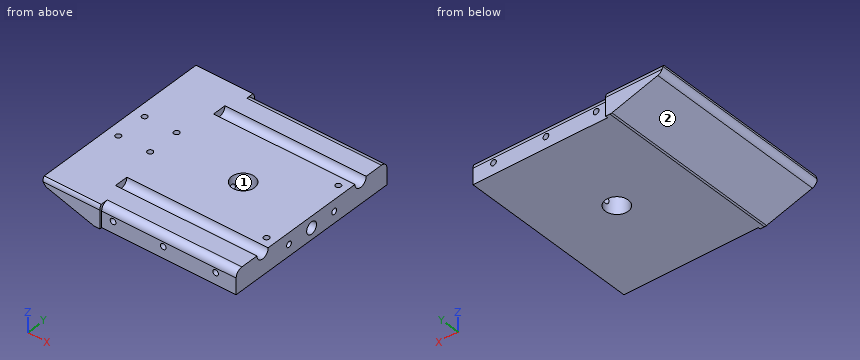
```python
from build123d import *

# Parameters (mm, degrees)
CYLINDER284_R          = 3
CYLINDER284_DEPTH      = 62
CYLINDER285_R          = 3
CYLINDER285_DEPTH      = 62
CYLINDER280_R          = 1.2
CYLINDER280_DEPTH      = 4
CYLINDER281_R          = 1.2
CYLINDER281_DEPTH      = 4
CYLINDER282_R          = 1.2
CYLINDER282_DEPTH      = 8
CYLINDER283_R          = 1.2
CYLINDER283_DEPTH      = 8
CYLINDER453_R          = 1.2
CYLINDER453_DEPTH      = 4
CYLINDER452_R          = 1.2
CYLINDER452_DEPTH      = 4
CYLINDER457_R          = 1.25
CYLINDER457_DEPTH      = 15
CYLINDER456_R          = 1.25
CYLINDER456_DEPTH      = 15
BOX301_W               = 25
BOX301_H               = 82
BOX301_DEPTH           = 1
CYLINDER278_R          = 1.25
CYLINDER278_DEPTH      = 15
CYLINDER277_R          = 1.25
CYLINDER277_DEPTH      = 15
CYLINDER279_R          = 1.25
CYLINDER279_DEPTH      = 15
CYLINDER272_R          = 1.6
CYLINDER272_DEPTH      = 41
CYLINDER274_R          = 2.6
CYLINDER274_DEPTH      = 20
CYLINDER273_R          = 1.4
CYLINDER273_DEPTH      = 51
CYLINDER286_R          = 1.25
CYLINDER286_DEPTH      = 15
CYLINDER287_R          = 1.25
CYLINDER287_DEPTH      = 15
CYLINDER288_R          = 1.25
CYLINDER288_DEPTH      = 15
CYLINDER271_R          = 5
CYLINDER271_DEPTH      = 19
BOX215_W               = 30
BOX215_H               = 82
BOX215_DEPTH           = 10
BOX215_PLACEMENT_ANGLE = 17
BOX214_W               = 25
BOX214_H               = 62
BOX214_DEPTH           = 1.5
BOX213_W               = 25
BOX213_H               = 82
BOX213_DEPTH           = 11
FILLET085_R            = 3
BOX212_W               = 60
BOX212_H               = 80
BOX212_DEPTH           = 10
FILLET084_R            = 3
FILLET086_R            = 3


with BuildPart() as cylinder284:
    # Cylinder284 → Cylinder284 (new body)
    with BuildSketch(Plane(origin=(67, 5, 19), x_dir=(0, 0, -1), z_dir=(1, 0, 0))):
        Circle(CYLINDER284_R)
    extrude(amount=CYLINDER284_DEPTH)


with BuildPart() as fusion252:
    # Cylinder285 → Cylinder285 (new body)
    with BuildSketch(Plane(origin=(67, 57, 19), x_dir=(0, 0, -1), z_dir=(1, 0, 0))):
        Circle(CYLINDER285_R)
    extrude(amount=CYLINDER285_DEPTH)

    # Fusion252: union Cylinder284
    add(cylinder284.part)


with BuildPart() as cylinder280:
    # Cylinder280 → Cylinder280 (new body)
    with BuildSketch(Plane(origin=(50, 24, 15), x_dir=(1, 0, 0), z_dir=(0, 0, 1))):
        Circle(CYLINDER280_R)
    extrude(amount=CYLINDER280_DEPTH)


with BuildPart() as cylinder281:
    # Cylinder281 → Cylinder281 (new body)
    with BuildSketch(Plane(origin=(50, 38, 15), x_dir=(1, 0, 0), z_dir=(0, 0, 1))):
        Circle(CYLINDER281_R)
    extrude(amount=CYLINDER281_DEPTH)


with BuildPart() as cylinder282:
    # Cylinder282 → Cylinder282 (new body)
    with BuildSketch(Plane(origin=(64, 24, 11), x_dir=(1, 0, 0), z_dir=(0, 0, 1))):
        Circle(CYLINDER282_R)
    extrude(amount=CYLINDER282_DEPTH)


with BuildPart() as cylinder283:
    # Cylinder283 → Cylinder283 (new body)
    with BuildSketch(Plane(origin=(64, 38, 11), x_dir=(1, 0, 0), z_dir=(0, 0, 1))):
        Circle(CYLINDER283_R)
    extrude(amount=CYLINDER283_DEPTH)


with BuildPart() as cylinder453:
    # Cylinder453 → Cylinder453 (new body)
    with BuildSketch(Plane(origin=(125, 12, 15), x_dir=(1, 0, 0), z_dir=(0, 0, 1))):
        Circle(CYLINDER453_R)
    extrude(amount=CYLINDER453_DEPTH)


with BuildPart() as fusion406:
    # Cylinder452 → Cylinder452 (new body)
    with BuildSketch(Plane(origin=(125, 50, 15), x_dir=(1, 0, 0), z_dir=(0, 0, 1))):
        Circle(CYLINDER452_R)
    extrude(amount=CYLINDER452_DEPTH)

    # Fusion406: union Cylinder280, Cylinder281, Cylinder282, Cylinder283, Cylinder453
    add(cylinder280.part)
    add(cylinder281.part)
    add(cylinder282.part)
    add(cylinder283.part)
    add(cylinder453.part)


with BuildPart() as cylinder457:
    # Cylinder457 → Cylinder457 (new body)
    with BuildSketch(Plane(origin=(80, 43, 14), x_dir=(0, 0, -1), z_dir=(1, 0, 0))):
        Circle(CYLINDER457_R)
    extrude(amount=CYLINDER457_DEPTH)


with BuildPart() as fusion414:
    # Cylinder456 → Cylinder456 (new body)
    with BuildSketch(Plane(origin=(80, 19, 14), x_dir=(0, 0, -1), z_dir=(1, 0, 0))):
        Circle(CYLINDER456_R)
    extrude(amount=CYLINDER456_DEPTH)

    # Fusion413: union Cylinder457
    add(cylinder457.part)


with BuildPart() as fusion414_1:
    # Fusion413 placement: moved
    add(fusion414.part.moved(Location((34, 0, 0))))

    # Fusion414: union Fusion252, Fusion406
    add(fusion252.part)
    add(fusion406.part)


with BuildPart() as cube372:
    # Box301 → Box301 (new body)
    with BuildSketch(Plane(origin=(45, -10, 19), x_dir=(1, 0, 0), z_dir=(0, 0, 1))):
        with Locations((12.5, 41)):
            Rectangle(BOX301_W, BOX301_H)
    extrude(amount=BOX301_DEPTH)


with BuildPart() as cylinder278:
    # Cylinder278 → Cylinder278 (new body)
    with BuildSketch(Plane(origin=(6, 15, 14), x_dir=(1, 0, 0), z_dir=(0, -1, 0))):
        Circle(CYLINDER278_R)
    extrude(amount=CYLINDER278_DEPTH)


with BuildPart() as cylinder277:
    # Cylinder277 → Cylinder277 (new body)
    with BuildSketch(Plane(origin=(28, 15, 14), x_dir=(1, 0, 0), z_dir=(0, -1, 0))):
        Circle(CYLINDER277_R)
    extrude(amount=CYLINDER277_DEPTH)


with BuildPart() as fusion246:
    # Cylinder279 → Cylinder279 (new body)
    with BuildSketch(Plane(origin=(51, 15, 14), x_dir=(1, 0, 0), z_dir=(0, -1, 0))):
        Circle(CYLINDER279_R)
    extrude(amount=CYLINDER279_DEPTH)

    # Fusion246: union Cylinder278, Cylinder277
    add(cylinder278.part)
    add(cylinder277.part)


with BuildPart() as fusion246_1:
    # Fusion246 placement: moved
    add(fusion246.part.moved(Location((0, 56, 0))))


with BuildPart() as cylinder272:
    # Cylinder272 → Cylinder272 (new body)
    with BuildSketch(Plane(origin=(20, 31, 10), x_dir=(0, 0, -1), z_dir=(1, 0, 0))):
        Circle(CYLINDER272_R)
    extrude(amount=CYLINDER272_DEPTH)


with BuildPart() as cylinder274:
    # Cylinder274 → Cylinder274 (new body)
    with BuildSketch(Plane(origin=(41, 31, 10), x_dir=(0, 0, -1), z_dir=(1, 0, 0))):
        Circle(CYLINDER274_R)
    extrude(amount=CYLINDER274_DEPTH)


with BuildPart() as fusion249:
    # Cylinder273 → Cylinder273 (new body)
    with BuildSketch(Plane(origin=(10, 31, 10), x_dir=(0, 0, -1), z_dir=(1, 0, 0))):
        Circle(CYLINDER273_R)
    extrude(amount=CYLINDER273_DEPTH)

    # Fusion249: union Cylinder272, Cylinder274
    add(cylinder272.part)
    add(cylinder274.part)


with BuildPart() as fusion249_1:
    # Fusion249 placement: moved
    add(fusion249.part.moved(Location((-1, 0, 4))))


with BuildPart() as cylinder286:
    # Cylinder286 → Cylinder286 (new body)
    with BuildSketch(Plane(origin=(6, 15, 14), x_dir=(1, 0, 0), z_dir=(0, -1, 0))):
        Circle(CYLINDER286_R)
    extrude(amount=CYLINDER286_DEPTH)


with BuildPart() as cylinder287:
    # Cylinder287 → Cylinder287 (new body)
    with BuildSketch(Plane(origin=(28, 15, 14), x_dir=(1, 0, 0), z_dir=(0, -1, 0))):
        Circle(CYLINDER287_R)
    extrude(amount=CYLINDER287_DEPTH)


with BuildPart() as fusion254:
    # Cylinder288 → Cylinder288 (new body)
    with BuildSketch(Plane(origin=(51, 15, 14), x_dir=(1, 0, 0), z_dir=(0, -1, 0))):
        Circle(CYLINDER288_R)
    extrude(amount=CYLINDER288_DEPTH)

    # Fusion254: union Cylinder286, Cylinder287
    add(cylinder286.part)
    add(cylinder287.part)


with BuildPart() as fusion254_1:
    # Fusion254 placement: moved
    add(fusion254.part.moved(Location((0, -9, 0))))


with BuildPart() as fusion255:
    # Cylinder271 → Cylinder271 (new body)
    with BuildSketch(Plane(origin=(30, 31, 6), x_dir=(1, 0, 0), z_dir=(0, 0, 1))):
        Circle(CYLINDER271_R)
    extrude(amount=CYLINDER271_DEPTH)

    # Fusion255: union Fusion246, Fusion249, Fusion254
    add(fusion246_1.part)
    add(fusion249_1.part)
    add(fusion254_1.part)


with BuildPart() as cube295:
    # Box215 → Box215 (new body)
    with BuildSketch(Plane.XY):
        with Locations((15, 41)):
            Rectangle(BOX215_W, BOX215_H)
    extrude(amount=BOX215_DEPTH)


with BuildPart() as cube295_1:
    # Box215 placement: moved
    add(cube295.part.moved(Location((-29, -10, 7))).rotate(Axis((-29, -10, 7), (0, 1, 0)), BOX215_PLACEMENT_ANGLE))


with BuildPart() as cube294:
    # Box214 → Box214 (new body)
    with BuildSketch(Plane(origin=(-24, 0, 19), x_dir=(1, 0, 0), z_dir=(0, 0, 1))):
        with Locations((12.5, 31)):
            Rectangle(BOX214_W, BOX214_H)
    extrude(amount=BOX214_DEPTH)


with BuildPart() as fillet085:
    # Box213 → Box213 (new body)
    with BuildSketch(Plane(origin=(-24, -10, 9), x_dir=(1, 0, 0), z_dir=(0, 0, 1))):
        with Locations((12.5, 41)):
            Rectangle(BOX213_W, BOX213_H)
    extrude(amount=BOX213_DEPTH)

    # Cut222: cut Cube294
    add(cube294.part, mode=Mode.SUBTRACT)

    # Fillet085
    fillet085_edges = [fillet085.edges().sort_by_distance(p)[0] for p in [
        (-11.5, -10, 20),
        (-11.5, 72, 20),
    ]]
    fillet(fillet085_edges, radius=FILLET085_R)


with BuildPart() as fifth_wheel_plate_wide:
    # Box212 → Box212 (new body)
    with BuildSketch(Plane(origin=(0, -9, 9), x_dir=(1, 0, 0), z_dir=(0, 0, 1))):
        with Locations((30, 40)):
            Rectangle(BOX212_W, BOX212_H)
    extrude(amount=BOX212_DEPTH)

    # Fillet084
    fillet084_edges = [fifth_wheel_plate_wide.edges().sort_by_distance(p)[0] for p in [
        (30, -9, 19),
        (30, 71, 19),
    ]]
    fillet(fillet084_edges, radius=FILLET084_R)

    # Fusion253: union Fillet085
    add(fillet085.part)

    # Cut223: cut Cube295
    add(cube295_1.part, mode=Mode.SUBTRACT)

    # Cut224: cut Fusion255
    add(fusion255.part, mode=Mode.SUBTRACT)


with BuildPart() as fifth_wheel_plate_wide_1:
    # Cut224 placement: moved
    add(fifth_wheel_plate_wide.part.moved(Location((69, 0, 0))))

    # Fillet086
    fillet086_edges = [fifth_wheel_plate_wide_1.edges().sort_by_distance(p)[0] for p in [
        (67.661331, 31, 9),
        (45, 31, 15.928264),
    ]]
    fillet(fillet086_edges, radius=FILLET086_R)

    # Cut299: cut Cube372
    add(cube372.part, mode=Mode.SUBTRACT)

    # Cut304: cut Fusion414
    add(fusion414_1.part, mode=Mode.SUBTRACT)


solid = fifth_wheel_plate_wide_1.part
```
Can you work these out from the model? Positions are in its coordinate system, mm. Face numbers are marked on the shaded views. Coordinates: 2 decimals unless noted, no trailing zeros. Loops run counter-clockwise (first coordinate to the right, second up) from the corner with the lowest first, then second, coordinate; pieces in that order, holes last. Notation, with made-up numbers: (11, 84) -> (21, 84) arc R21 cw to (21, 102) -> close; hole circle Ø10 at (18, 75). An arc over 180 degrees is marked (long way). Put each result on its own line as item: value. Start each with the question number.
Q1. I want a section at C-C (y = 19). Write out the boundary of the cut face in (x, z).
Q2. I'm going to push flat-ended pins straight in: P1, Ø3, axis at x = 65, y = 62.5, coming from the -Z side; P2, Ø3, axis at x = 120, z = 14, coming from the -Y side; P3, Ø2, axis at x = 120, z = 14, coming from the +Y side. Where does each tip first touch, or does it pass through?
Q3. I want a section at A-A (y = 57). Write out the boundary of the cut face in (x, z), plus the area to 3 significant figures.
Q4. If I drill on line 1 (Z direction, x = 84, y = 31); line 2 (Y direction, x = 64, z = 16.25); line 3 (Y direction, x = 87, z = 17.25), over which ranges is the centre line in solid material (lowest first)? Write a range as [from, to].
Q5. I want a section at B-B (x = 125). Write out the boundary of the cut face in (y, z).
Q6. I want a section at D-D (x = 83). Write out the boundary of the cut face in (y, z), plus the area to 3 significant figures.
Q7. Thinking about a two-plate mould opening in Y: for the marked faces 1 and 2, which applies, pulls with the +Y half, pulls with the -Y half, needs draft (parallel to the pull), parting line crosses it, or undercut?
Taken from the geometry:
1. outline: (45, 18.15) arc R3 ccw to (47.12, 15.28) -> (67.23, 9.13) arc R3 ccw to (68.11, 9) -> (129, 9) -> (129, 12.75) -> (114, 12.75) -> (114, 15.25) -> (129, 15.25) -> (129, 19) -> (45, 19) -> close
2. P1: stops at z = 9.36
2. P2: stops at y = -9
2. P3: stops at y = 56
3. outline: (45, 18.15) arc R3 ccw to (47.12, 15.28) -> (67.23, 9.13) arc R3 ccw to (68.11, 9) -> (129, 9) -> (129, 16) -> (67, 16) -> (67, 19) -> (45, 19) -> close; hole circle Ø2.5 at (75, 14); hole circle Ø2.5 at (97, 14); hole circle Ø2.5 at (120, 14)
3. area: 560 mm2
4. line 1: z = [9, 12.6], [15.4, 19]
4. line 2: y = [-10, 22.8], [25.2, 36.8], [39.2, 72]
4. line 3: y = [-8.73, 2.56], [7.44, 54.56], [59.44, 70.73]
5. outline: (-9, 9) -> (71, 9) -> (71, 16) arc R3 ccw to (68, 19) -> (60, 19) arc R3 cw to (54, 19) -> (51.2, 19) -> (51.2, 15) -> (48.8, 15) -> (48.8, 19) -> (13.2, 19) -> (13.2, 15) -> (10.8, 15) -> (10.8, 19) -> (8, 19) arc R3 cw to (2, 19) -> (-6, 19) arc R3 ccw to (-9, 16) -> close; hole circle Ø2.5 at (19, 14); hole circle Ø5.2 at (31, 14); hole circle Ø2.5 at (43, 14)
6. outline: (-9, 9) -> (71, 9) -> (71, 16) arc R3 ccw to (68, 19) -> (60, 19) arc R3 cw to (54, 19) -> (8, 19) arc R3 cw to (2, 19) -> (-6, 19) arc R3 ccw to (-9, 16) -> close; hole circle Ø2.8 at (31, 14)
6. area: 762 mm2
7. face 1: undercut
7. face 2: needs draft
